Print and shaded views of the part. All mm, measured from the part's lowest x, y and z. A direction names the side the tool comes from. Round coordinates to 2 decimals unless told otherwise and drop trailing zeros. Loops run counter-clockwise (first coordinate to the right, second up) from the corner with the lowest first, then second, coordinate; pieces in that order, holes last. Notation, with made-up numbers: M -7.5,-22 L 46.5,-22 A28 cw 46.5,15 Z; hole C 27,69.5 d2. An arc over 180 degrees is marked long. One line per item, written item: value. Start each with the question number.
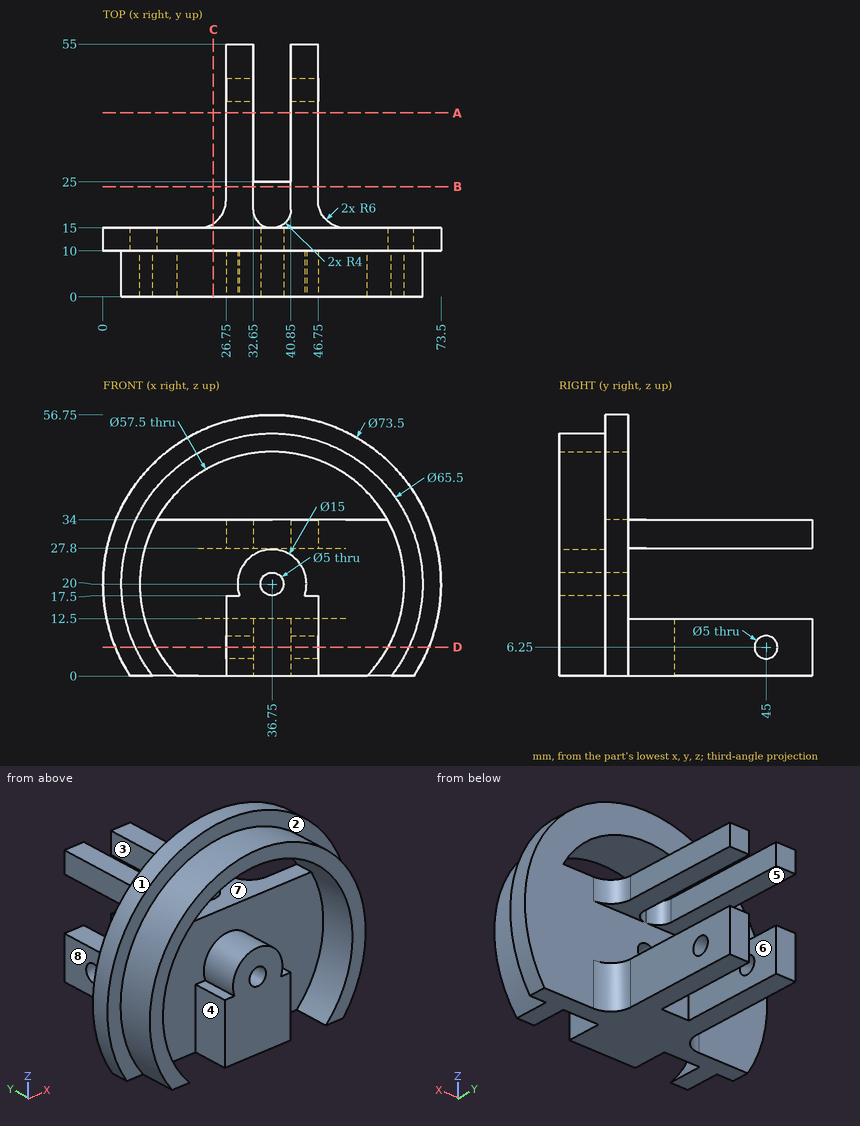
(1) Which spindle directions (+Z, -Z, +X, -X, +Y, -Y) get a long thin tool onto all of the face, cutting with end or side? Do the marked faces 4, 5, 6, 7 and 8. Say none if no direction does.
(2) Slice it at B-B, the plane y = 24. List the corners of the cut face in (x, z).
(3) Flat gauge pins, fed straight in: P1, Ø6, axis at y = 19.5, z = 7.5, coming from the -X side; P2, Ø3, axis at y = 4, z = 5, coming from the -X side; P3, Ø1.9, axis at y = 39, z = 31, coming from the -X side; P4, Ø8, axis at x = 33, z = 18, coming from the -Y side. Where does each tip first touch, or does it go through?
(4) Slice it at C-C, the plane x = 24. List the corners of the cut face in (y, z).
(5) Probe L1, parallel to X at y = 9, z = 20; L2, parallel to Y at x = 43.75, z = 6.25; L3, parallel to Z at x = 29, y = 29. List the from-to ranges inside material, lowest first.
(6) Mould opens along X. For the marked faces 1, 2 and 3 say: pulls with the +X half, pulls with the -X half, needs draft (parallel to the pull), parting line crosses it, or undercut.
(7) Slice it at D-D, the plane z = 6.25. Count the separate pieces of the cut face and the enclosed holes in it, and give its area (3 significant figures).
(8) Slice it at A-A, the plane y = 40. List the corners of the cut face in (x, z).
Check result:
1. face 4: -Z, -Y
1. face 5: +X, -X, +Y
1. face 6: +Z, -Z, +Y
1. face 7: +Y, -Y
1. face 8: +Z, -Z, -X, +Y
2. outline: M 26.75,0 L 46.75,0 L 46.75,12.5 L 26.75,12.5 Z; M 26.75,27.8 L 32.65,27.8 L 32.65,34 L 26.75,34 Z; M 40.85,27.8 L 46.75,27.8 L 46.75,34 L 40.85,34 Z
3. P1: stops at x = 24.72
3. P2: stops at x = 6.91
3. P3: stops at x = 26.75
3. P4: stops at y = 0
4. outline: M 0,45.77 L 15,45.77 L 15,54.47 L 10,54.47 L 10,50.17 L 0,50.17 Z; M 10,0 L 15.96,0 L 15.96,12.5 L 15,12.5 L 15,27.8 L 15.96,27.8 L 15.96,34 L 10,34 Z
5. L1: x = 4 to 8, 29.25 to 34.25, 39.25 to 44.25, 65.5 to 69.5
5. L2: y = 0 to 42.5, 47.5 to 55
5. L3: z = 0 to 12.5, 27.8 to 34
6. face 1: parting line crosses it
6. face 2: needs draft
6. face 3: undercut
7. separate pieces: 3
7. enclosed holes: 0
7. area: 1,140 mm^2
8. outline: M 26.75,0 L 32.65,0 L 32.65,12.5 L 26.75,12.5 Z; M 26.75,27.8 L 32.65,27.8 L 32.65,34 L 26.75,34 Z; M 40.85,0 L 46.75,0 L 46.75,12.5 L 40.85,12.5 Z; M 40.85,27.8 L 46.75,27.8 L 46.75,34 L 40.85,34 Z
